Geometry check sheet. Reference: drawing and pictorial views, mm from the part's lowest x, y, z. A direction names the side the tool comes from. Coordinates: 2 decimals unless noted, no trailing zeros. Write each loop counter-clockwise with the first axis right and the second up, starting at its lowest first coordinate (ties: lowest second). Pieces come first, ordered by that corner, then holes. Notation, with made-up numbers: M 87.5,7.5 L 120.5,7.5 A23 ccw 120.5,38.5 Z; hole C 55,-20.75 d10. An arc over 180 degrees is marked long. One line per item, written item: value.
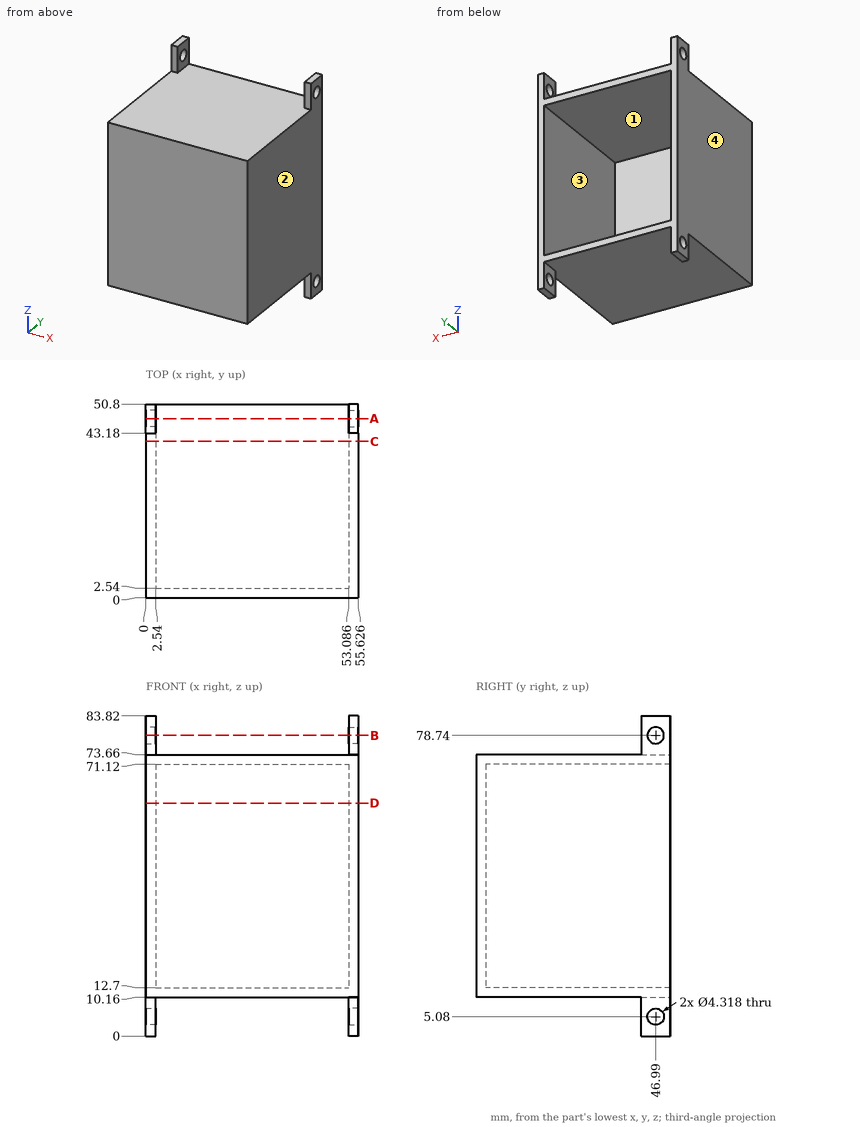
Item 1: Access from +Z, -Z, +X, -X, +Y, -Y to the whole of each face (thin tool, end or side, straight path). Record for the marked faces 3 and 4.
The answers:
face 3: +Y
face 4: +Z, -Z, -X, +Y, -Y
Item 2: Draft check along Z on the marked faces 1 and 2. Enter one of: released by +Z, released by -Z, zero draft, split by the parting line, or undercut.
The answers:
face 1: undercut
face 2: zero draft
Item 3: Cross-section at B-B, the plane z = 78.74. Enter the section's corners in (x, y).
The answers:
outline: M 0,43.18 L 2.54,43.18 L 2.54,44.83 L 0,44.83 Z; M 0,49.15 L 2.54,49.15 L 2.54,50.8 L 0,50.8 Z; M 53.09,43.18 L 55.63,43.18 L 55.63,44.83 L 53.09,44.83 Z; M 53.09,49.15 L 55.63,49.15 L 55.63,50.8 L 53.09,50.8 Z
Item 4: Go/stop test with flat-tipped pins: P1, Ø4, axis at x = 33.5, y = 27, coming from the -Z side; P2, Ø14.5, axis at y = 31.5, z = 40, coming from the -X side; P3, Ø5, axis at x = 18.5, y = 13.5, coming from the +Z side; P4, Ø2, axis at x = 2, z = 7, coming from the -Y side. Record where each tip stops, or that it passes through.
The answers:
P1: stops at z = 10.16
P2: stops at x = 0
P3: stops at z = 73.66
P4: stops at y = 43.18
Item 5: Cross-section at A-A, the plane y = 46.99. Give the number of separate pieces and of enclosed holes in the cut face, and give its area (3 significant figures).
The answers:
separate pieces: 5
enclosed holes: 1
area: 639 mm²
Item 6: Cross-section at C-C, the plane y = 41. Enter the section's corners in (x, z).
The answers:
outline: M 0,10.16 L 55.63,10.16 L 55.63,73.66 L 0,73.66 Z; hole M 2.54,12.7 L 53.09,12.7 L 53.09,71.12 L 2.54,71.12 Z
Item 7: Cross-section at D-D, the plane z = 61. Enter the section's corners in (x, y).
The answers:
outline: M 0,0 L 55.63,0 L 55.63,50.8 L 53.09,50.8 L 53.09,2.54 L 2.54,2.54 L 2.54,50.8 L 0,50.8 Z
Item 8: Scan lines: line 1 (Z direction, x = 0.6, y = 46.99); line 2 (X direction, y = 49, z = 13); line 3 (Z direction, x = 41.5, y = 11). Record each from-to range of solid material in increasing order.
The answers:
line 1: z = 0 to 2.92, 7.24 to 76.58, 80.9 to 83.82
line 2: x = 0 to 2.54, 53.09 to 55.63
line 3: z = 10.16 to 12.7, 71.12 to 73.66
